Study the drawing (mm; zero at the part's minimum x, y, z) and answer. Round coordinates to 2 decimals unless told otherwise and drop trailing zeros. Write each loop counter-clockwise with the first axis right and the second up, starting at its lowest first coordinate (ties: lowest second). Pieces come first, ordered by that corner, then holes. Notation, with made-up numbers: (58, 78.25) - (103, 78.25) arc R18 ccw to (103, 97.25) - close; hole circle Ø10 at (87.25, -32). An arc over 180 degrees is marked (long way). Use one line per item in the form item = value. Start each with the question number.
1) For a pull along X with two mould halves and no side action, classify the marked faces 1, 2 and 3 as released by +X, released by -X, zero draft, split by the parting line, or undercut.
2) The part is cut by section A-A, the plane z = 1.75. Give the vertices of the cut face in (x, y) (1 decimal).
3) Each of these flat-tipped pins is pushed along its axis until it touches: pin 1 (12.5 mm diameter, centred on x = 12, y = 13.86, fed in from +Z); pin 2 (2 mm diameter, centred on y = 22.5, z = 6.5, fed in from -X). Where does it stop, or does it pass through?
4) Consider line 1 along X through (y, z) = (9.5, 6.5) (1 decimal); line 2 along X through (y, z) = (18.25, 4) (1 decimal); line 3 along X through (y, z) = (21.25, 7) (1 decimal). Determine where each line is inside the solid, lowest interval first. Write a range as from..to.
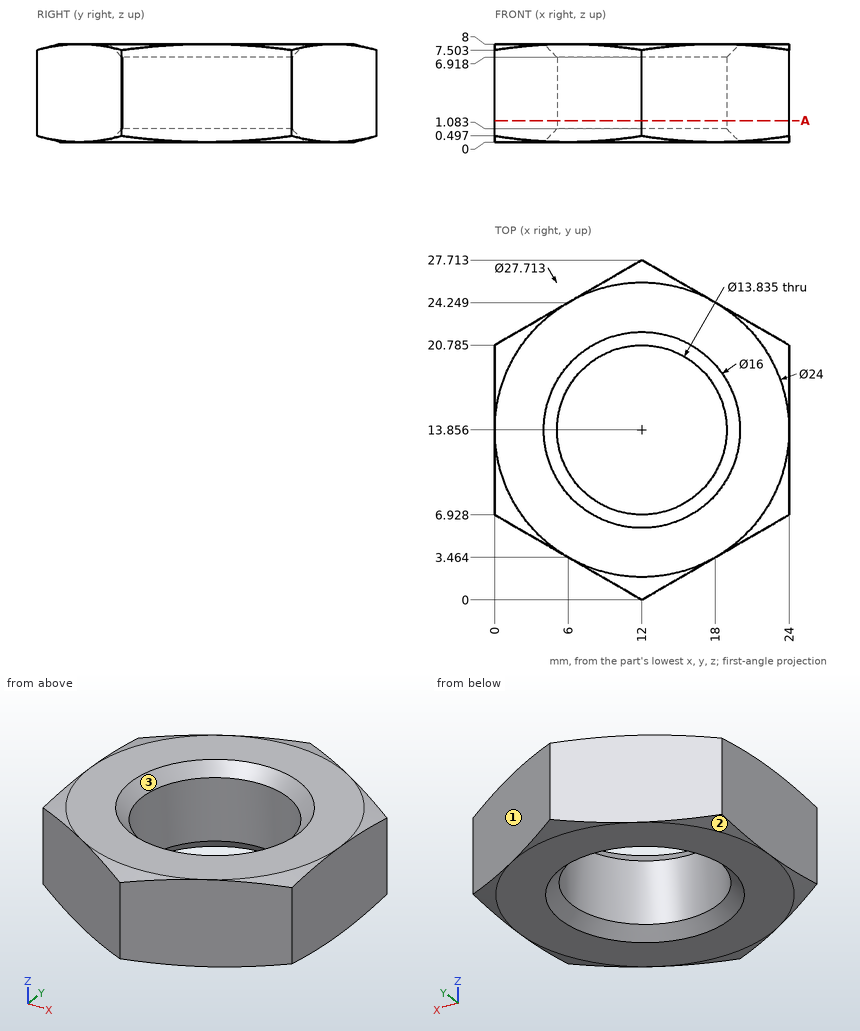
Geometry results:
q1.face_1 = released by +X
q1.face_2 = released by -X
q1.face_3 = undercut
q2.outline = (0, 6.9) - (12, 0) - (24, 6.9) - (24, 20.8) - (12, 27.7) - (0, 20.8) - close; hole circle Ø13.8 at (12, 13.9)
q3.pin_1 = through
q3.pin_2 = 1.24
q4.line_1 = 0..6.6, 17.4..24
q4.line_2 = 0..6.7, 17.3..24
q4.line_3 = 0.8..23.2
